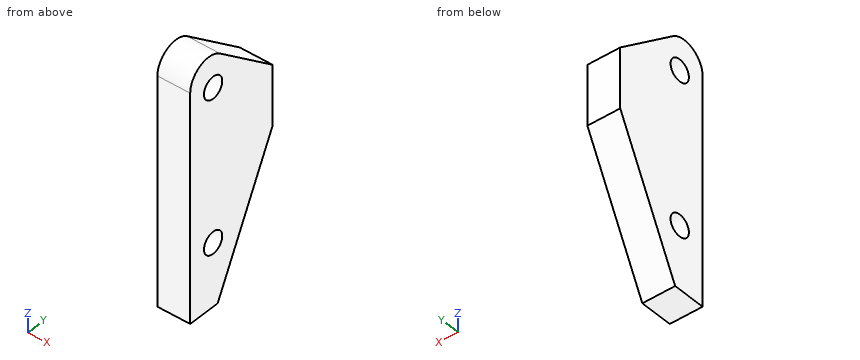
Autodesk Inventor part; units mm, degrees
ref_plane "YZ Plane" through (0, 0, 0) normal (1, 0, 0) x (0, 1, 0)
ref_plane "XZ Plane" through (0, 0, 0) normal (0, 1, 0) x (-1, 0, 0)
ref_plane "XY Plane" through (0, 0, 0) normal (0, 0, 1) x (1, 0, 0)
sketch "Base" plane through (0, 0, 0) normal (1, 0, 0) x (0, 1, 0)
  line L0 (3, -25) -> (0, -25)
  line L1 (3, -25) -> (9, -12.6982)
  line L2 (9, -12.6982) -> (9, -7.1982)
  line L3 (9, -7.1982) -> (0, 0)
  line L4 (0, -25) -> (0, 0)
  dimension "d0" = 9
  dimension "d2" = 26
  dimension "d3" = 25
  dimension "d4" = 3
  dimension "d24" = 5.5
extrude "BaseFeature" add sketch "Base" along normal blind 3
fillet "BaseFilletsFeature" radius 2 1 edges at (1.5, 0, 0)
sketch "BaseHoles" plane through (0, 0, 0) normal (-1, 0, 0) x (0, 0, 1)
  line L0 (-25, 2.5) -> (-2.2241, 2.5) construction
  line L1 (-2.5987, 3.2492) -> (-7.1982, 9) construction
  circle A0 centre (-19.2241, 2.5) radius 1.75
  circle A1 centre (-5.2241, 2.5) radius 1.75
  line L2 (-4.1606, 0) -> (-25, 0)
  arc A2 (-4.1606, 0) -> (-2.5987, 3.2492) centre (-4.1606, 2) ccw
  line L3 (-25, 0) -> (-25, 3)
  dimension "d9" = 3.5
  dimension "d12" = 3
  dimension "d23" = 14
  dimension "d25" = 2.5
hole "BaseHolesFeature" at (0, 2.5, -19.2241) at (0, 2.5, -5.2241) direction (1, 0, 0) diameter 2 end through all
properties part number "Knuckle"
The listing builds one solid part. Answer for the finished solid, in the listing's coordinates (mm). Coordinates: 2 decimals unless noted, no trailing zeros. Write each loop counter-clockwise with the first axis right and the second up, starting at its lowest first coordinate (ties: lowest second). Pieces come first, ordered by that corner, then holes. Notation, with made-up numbers: (-40, -19) - (0, -19) arc R7 ccw to (0, -6) - close; hole circle Ø8 at (36, -38). An arc over 180 degrees is marked (long way). Return JSON: item names as keys, results as strings. Group by question number.
Q1. The part is cut by section D-D on y = 5.25. Write down the section's boundary in (x, z), and give its area (3 significant figures).
Q2. The part is cut by section B-B on x = 2.25. Write down the section's boundary in (y, z).
Q3. Find the intervals of material crossed by line 1 along Z through (x, y) = (2.25, 2.5); line 2 along Z through (x, y) = (1.65, 3.25); line 3 along Y through (x, z) = (1.85, -19.5), in increasing order. Write a range as [from, to].
Q4. A flat-ended cylindrical pin translates along its axis: pin 1 Ø1.5 at (x, y) = (2, 3) entering from +Z. Find the tip coordinate at first contact, or state that the pin passes through.
Q5. The part is cut by section A-A on y = 2.75. Write down the section's boundary in (x, z).
Q6. The part is cut by section C-C on z = -20. Write down the section's boundary in (x, y), and give its area (3 significant figures).
Evaluation:
{
 "1": {"outline": "(0, -20.39) - (3, -20.39) - (3, -4.2) - (0, -4.2) - close", "area": "48.6 mm2"},
 "2": {"outline": "(0, -25) - (3, -25) - (9, -12.7) - (9, -7.2) - (3.25, -2.6) arc R2 ccw to (0, -4.16) - close; hole circle Ø2 at (2.5, -19.22); hole circle Ø2 at (2.5, -5.22)"},
 "3": {"line 1": "z = [-25, -20.22], [-18.22, -6.22], [-4.22, -2.22]", "line 2": "z = [-24.49, -19.89], [-18.56, -5.89], [-4.56, -2.6]", "line 3": "y = [0, 1.54], [3.46, 5.68]"},
 "4": {"pin 1": "stops at z = -2.18"},
 "5": {"outline": "(0, -25) - (3, -25) - (3, -20.19) - (0, -20.19) - close; (0, -18.26) - (3, -18.26) - (3, -6.19) - (0, -6.19) - close; (0, -4.26) - (3, -4.26) - (3, -2.31) - (0, -2.31) - close"},
 "6": {"outline": "(0, 0) - (3, 0) - (3, 1.87) - (0, 1.87) - close; (0, 3.13) - (3, 3.13) - (3, 5.44) - (0, 5.44) - close", "area": "12.5 mm2"}
}
